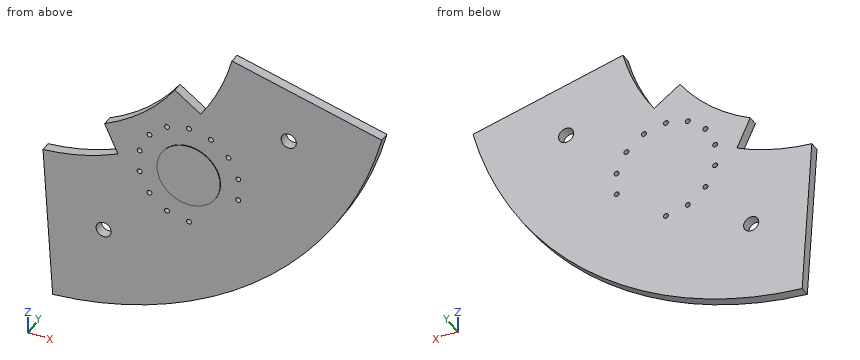
from build123d import *

# Parameters (mm, degrees)
SKETCH2_R           = 5
BOSS_EXTRUDE1_DEPTH = 1.6
SKETCH3_R           = 1.2
CUT_EXTRUDE1_DEPTH  = 1.7
SKETCH10_R          = 0.39
CUT_EXTRUDE6_DEPTH  = 10
BOSS_EXTRUDE3_START = -1.7
SKETCH11_R          = 5
BOSS_EXTRUDE3_DEPTH = 1.7


with BuildPart() as part:
    # Sketch2 → Boss-Extrude1 (new body)
    with BuildSketch(Plane(origin=(0, 0, 0), x_dir=(1, 0, 0), z_dir=(0, 1, 0))):
        with BuildLine():
            Line((-12.84928634, 13.429675326), (-14.381752422, -11.022350105))
            ThreePointArc((-14.381752422, -11.022350105), (-8.311058851, -11.976103518), (-2.52245469, -14.038875409))
            Line((-2.52245469, -14.038875409), (-4.632066163, -18.572035393))
            ThreePointArc((-4.632066163, -18.572035393), (1.543927211, -22.501579223), (6.490366829, -27.897591081))
            Line((6.490366829, -27.897591081), (10.586127051, -25.029708899))
            ThreePointArc((10.586127051, -25.029708899), (13.540412509, -30.180153963), (15.523932384, -35.776629267))
            Line((15.523932384, -35.776629267), (39.259103853, -29.702780788))
            ThreePointArc((39.259103853, -29.702780788), (20.218425809, 0.336488596), (-12.84928634, 13.429675326))
        make_face()
        with Locations(Location((8.721864443, -13.940574544, 0), (0, 0, 270))):
            Circle(SKETCH2_R, mode=Mode.SUBTRACT)
    extrude(amount=BOSS_EXTRUDE1_DEPTH)

    # Sketch3 → Cut-Extrude1 (cut)
    with BuildSketch(Plane(origin=(0, 1.6, 0), x_dir=(1, 0, 0), z_dir=(0, 1, 0))):
        with Locations(Location((-4.780794064, -0.288914882, 0), (0, 0, 270))):
            Circle(SKETCH3_R)
        with Locations(Location((24.519221563, -24.855385868, 0), (0, 0, 270))):
            Circle(SKETCH3_R)
    extrude(amount=-CUT_EXTRUDE1_DEPTH, mode=Mode.SUBTRACT)

    # Sketch10 → Cut-Extrude6 (cut)
    with BuildSketch(Plane(origin=(0, 1.6, 0), x_dir=(1, 0, 0), z_dir=(0, 1, 0))):
        with Locations(Location((5.25079453, -6.732823601, 0), (0, 0, 270))):
            Circle(SKETCH10_R)
        with Locations(Location((8.721864443, -5.940574544, 0), (0, 0, 270))):
            Circle(SKETCH10_R)
        with Locations(Location((2.467212583, -8.952656129, 0), (0, 0, 270))):
            Circle(SKETCH10_R)
        with Locations(Location((0.922441145, -12.160407072, 0), (0, 0, 270))):
            Circle(SKETCH10_R)
        with Locations(Location((0.922441145, -15.720742016, 0), (0, 0, 270))):
            Circle(SKETCH10_R)
        with Locations(Location((2.467212583, -18.928492959, 0), (0, 0, 270))):
            Circle(SKETCH10_R)
        with Locations(Location((5.25079453, -21.148325487, 0), (0, 0, 270))):
            Circle(SKETCH10_R)
        with Locations(Location((8.721864443, -21.940574544, 0), (0, 0, 270))):
            Circle(SKETCH10_R)
        with Locations(Location((12.192934355, -21.148325487, 0), (0, 0, 270))):
            Circle(SKETCH10_R)
        with Locations(Location((14.976516302, -18.928492959, 0), (0, 0, 270))):
            Circle(SKETCH10_R)
        with Locations(Location((16.52128774, -15.720742016, 0), (0, 0, 270))):
            Circle(SKETCH10_R)
        with Locations(Location((16.52128774, -12.160407072, 0), (0, 0, 270))):
            Circle(SKETCH10_R)
    extrude(amount=-CUT_EXTRUDE6_DEPTH, mode=Mode.SUBTRACT)

    # Sketch11 → Boss-Extrude3 (add)
    with BuildSketch(Plane(origin=(0, 1.6, 0), x_dir=(1, 0, 0), z_dir=(0, 1, 0)).offset(BOSS_EXTRUDE3_START)):
        with Locations(Location((8.721864443, -13.940574544, 0), (0, 0, 270))):
            Circle(SKETCH11_R)
    extrude(amount=BOSS_EXTRUDE3_DEPTH)


solid = part.part
For this review, take the finished solid that the model builds, in its own axes (mm). Coordinates: 2 decimals unless noted, no trailing zeros. Loops run counter-clockwise (first coordinate to the right, second up) from the corner with the lowest first, then second, coordinate; pieces in that order, holes last. Notation, with made-up numbers: (50, 75) - (106, 75) arc R24 cw to (106, 113) - close; hole circle Ø3 at (-2.5, 30.25). An arc over 180 degrees is marked (long way). Use a Markdown table: item, result. Add a question column.
Item 1: We need section A-A (y = 0.75). Give the number of separate pieces and of enclosed holes in the cut face, and give its area (3 significant figures).
Item 2: For line 1 (Y direction, x = 30.5, z = 13); line 2 (X direction, y = 1.4, z = 0.5); line 3 (X direction, y = 0.35, z = 24.5), list the stretches that pass through material, from the lowest coordinate up.
Item 3: We need section B-B (x = 21.5). Give the boundary of the cut face in (y, z), and give its area (3 significant figures).
Item 4: Insertion check: pin 1 Ø5 at (x, z) = (31.5, 6) entering from -Y; pin 2 Ø3 at (x, z) = (24.52, 24.86) entering from -Y. Each pin has a flat end and moves straight along its axis. Give the tip position at first contact, or say it passes through.
Item 5: We need section C-C (z = 29). Give the boundary of the cut face in (x, y), and give its area (3 significant figures).
Results list:
| question | item | result |
|---|---|---|
| 1 | separate pieces | 1 |
| 1 | enclosed holes | 14 |
| 1 | area | 1,460 mm^2 |
| 2 | line 1 | y = 0 to 1.6 |
| 2 | line 2 | x = -13.72 to -5.96, -3.6 to 21.21 |
| 2 | line 3 | x = 3.69 to 23.37, 25.67 to 37.66 |
| 3 | outline | (0, 0.76) - (1.6, 0.76) - (1.6, 34.25) - (0, 34.25) - close |
| 3 | area | 53.6 mm^2 |
| 4 | pin 1 | passes through |
| 4 | pin 2 | stops at y = 0 |
| 5 | outline | (12.97, 0) - (39.07, 0) - (39.07, 1.6) - (12.97, 1.6) - close |
| 5 | area | 41.8 mm^2 |
